Check sheet for the modelled part. Datum: model origin and axes. Units: mm. Face numbers are marked on the shaded views. A direction names the side the tool comes from. Round coordinates to 2 decimals unless told otherwise and drop trailing zeros. Write each loop counter-clockwise with the first axis right and the second up, starting at its lowest first coordinate (ties: lowest second). Pieces come first, ordered by that corner, then holes. Notation, with made-up numbers: (12.5, 72.25) - (67.5, 72.25) arc R36 cw to (67.5, 110.25) - close; hole circle Ø10 at (2.25, -38). An arc over 180 degrees is marked (long way). Answer as a JSON object with one key per item and string values. Group by question number.
Item 1: Sectioned sample at D-D on y = -5.25. Record the boundary of the cut face in (x, z).
Item 2: Set-up check for the marked faces 1 and 2: record each of +Z, -Z, +X, -X, +Y, -Y from which the full face is reachable in a straight line by a thin tool's end or side.
Item 3: Sectioned sample at A-A on z = 0. Record the boundary of the cut face in (x, y), plus the area to 3 significant figures.
Item 4: Sectioned sample at C-C on y = -2. Record the boundary of the cut face in (x, z), plus the area to 3 significant figures.
Item 5: Gauge pin test, flat ends, axial feed: P1, Ø1, axis at x = -0.5, y = -7.5, coming from the +Z side; P2, Ø8, axis at x = -4.5, y = -3.5, coming from the -Z side; P3, Ø8, axis at y = -8, z = -6, coming from the -X side. Record the tip position at first contact, or that the pin passes through.
Item 6: Sectioned sample at B-B on x = 0. Record the boundary of the cut face in (y, z), plus the area to 3 significant figures.
Item 7: Thickness scan on line 1 (Y direction, x = -4.5, z = 5.25); line 2 (X direction, y = -4.5, z = -5.25); line 3 (Z direction, x = -4, y = -3.75). Record the ranges inside material, lowest first.
```python
from build123d import *

# Parameters (mm, degrees)
F0_R     = 8
F0_R_2   = 6.75
F0_R_3   = 5.515498
F1_DEPTH = 4.3
F4_R     = 0.5


with BuildPart() as f1:
    # F0 (on Front) → F1 (new body)
    with BuildSketch(Plane.XZ):
        Circle(F0_R)
        Circle(F0_R_2, mode=Mode.SUBTRACT)
        Circle(F0_R_2)
        Circle(F0_R_3, mode=Mode.SUBTRACT)
        Circle(F0_R_3)
    extrude(amount=F1_DEPTH)

    # F2 (on Right) → F3 (revolve)
    with BuildSketch(Plane.YZ):
        Polygon((-15.9, 0), (0, 0), (0, 6), (-4.3, 6), (-15.9, 5.5), align=None)
    revolve(axis=Axis((0, -7.95, 0), (0, 1, 0)))

    # F4
    f4_edges = [f1.edges().sort_by_distance(p)[0] for p in [
        (0, -15.9, -5.5),
        (-8, -4.3, 0),
    ]]
    fillet(f4_edges, radius=F4_R)


solid = f1.part
```
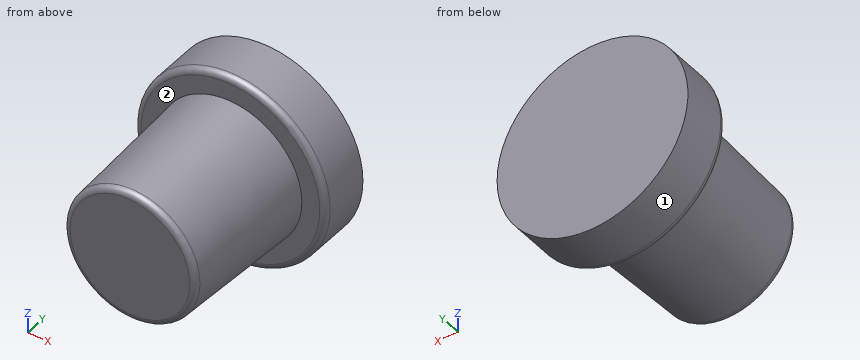
Completed:
{
 "1": {"outline": "circle Ø11.92 at (0, 0)"},
 "2": {"face 1": "+Y, -Y", "face 2": "-Y"},
 "3": {"outline": "(-8, -3.8) arc R0.5 ccw to (-7.5, -4.3) - (-6, -4.3) - (-5.52, -15.42) arc R0.5 ccw to (-5.02, -15.9) - (5.02, -15.9) arc R0.5 ccw to (5.52, -15.42) - (6, -4.3) - (7.5, -4.3) arc R0.5 ccw to (8, -3.8) - (8, 0) - (-8, 0) - close", "area": "202 mm²"},
 "4": {"outline": "circle Ø16 at (0, 0)", "area": "201 mm²"},
 "5": {"P1": "z = 5.88", "P2": "z = -7.98", "P3": "x = -6.2"},
 "6": {"outline": "(-15.9, -5.02) arc R0.5 ccw to (-15.42, -5.52) - (-4.3, -6) - (-4.3, -7.5) arc R0.5 ccw to (-3.8, -8) - (0, -8) - (0, 8) - (-3.8, 8) arc R0.5 ccw to (-4.3, 7.5) - (-4.3, 6) - (-15.42, 5.52) arc R0.5 ccw to (-15.9, 5.02) - close", "area": "202 mm²"},
 "7": {"line 1": "-4.3 to 0", "line 2": "-2.89 to 2.89", "line 3": "-6.93 to 6.93"}
}
